from build123d import *

# Parameters (mm, degrees)
BOSS_EXTRUDE1_DEPTH = 7.62


with BuildPart() as part:
    # Sketch1 → Revolve1 (revolve)
    with BuildSketch(Plane.XY):
        Polygon((0, 1.778), (0, 2.54), (0.635, 2.54), (0.635, 2.032), (7.366, 2.032), (7.366, 2.54), (7.62, 2.54), (7.62, 1.778), (0.635, 1.778), (0.635, 0), (0, 0), align=None)
    revolve(axis=Axis((0, 0, 0), (1, 0, 0)))

    # Sketch3 → Boss-Extrude1 (add)
    with BuildSketch(Plane(origin=(0, 0, 0), x_dir=(0, 0, -1), z_dir=(1, 0, 0))):
        with BuildLine():
            Line((-1.524, 0.762), (-0.762, 0.762))
            Line((-0.762, 0.762), (-0.762, 1.524))
            ThreePointArc((-0.762, 1.524), (0, 2.286), (0.762, 1.524))
            Line((0.762, 1.524), (0.762, 0.762))
            Line((0.762, 0.762), (1.524, 0.762))
            ThreePointArc((1.524, 0.762), (2.286, 0), (1.524, -0.762))
            Line((1.524, -0.762), (0.762, -0.762))
            Line((0.762, -0.762), (0.762, -1.524))
            ThreePointArc((0.762, -1.524), (0, -2.286), (-0.762, -1.524))
            Line((-0.762, -1.524), (-0.762, -0.762))
            Line((-0.762, -0.762), (-1.524, -0.762))
            ThreePointArc((-1.524, -0.762), (-2.286, 0), (-1.524, 0.762))
        make_face()
    extrude(amount=-BOSS_EXTRUDE1_DEPTH)


solid = part.part
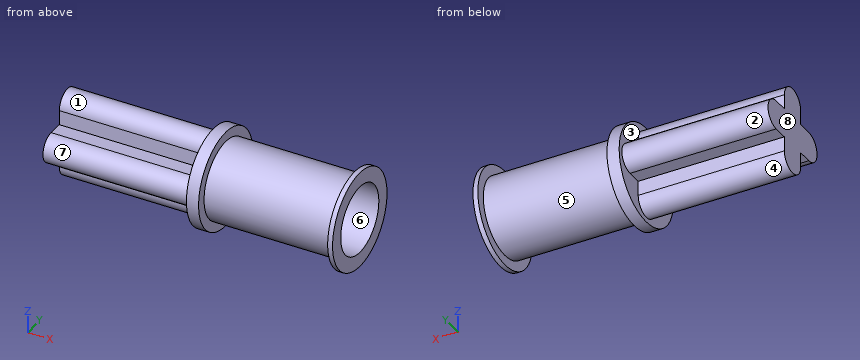
CAD build for the part. Positions are in the model's coordinates, mm. Face numbers are marked on the shaded views. A direction names the side the tool comes from. Round coordinates to 2 decimals unless told otherwise and drop trailing zeros. Write each loop counter-clockwise with the first axis right and the second up, starting at its lowest first coordinate (ties: lowest second). Pieces come first, ordered by that corner, then holes. Notation, with made-up numbers: M 55.25,54.25 L 75.25,54.25 A34 ccw 75.25,89.25 Z; hole C -17,7 d4. An arc over 180 degrees is marked long. Use a Markdown table: item, result. Add a question column.
1. Slice it at B-B on x = -4. Give the cut face in (y, z), then the cut area to 3 significant figures.
2. Slice it at D-D on x = 4. Give the cut face in (y, z), then the cut area to 3 significant figures.
3. Drill centre lines: probe 1 along X at (y, z) = (-2.15, 0.95) (3 decimals); probe 2 along Z at (x, y) = (-1.25, -1.1); probe 3 along X at (y, z) = (-0.7, -0.3) (3 decimals). Where is each one in solid material? Low to high.
4. 3-axis set-ups, long thin cutter, end or side, ignore diameter. For the marked faces 1, 2, 3, 4 and 5: which of +Z, -Z, +X, -X, +Y, -Y reach the whole face in a straight line?
5. Slice it at A-A on z = 0. Give the cut face in (x, y) (3 decimals).
6. Flat gauge pins, fed straight in: P1, Ø3, axis at x = 5, y = -1.5, coming from the -Z side; P2, Ø0.8, axis at x = -3.5, y = 1.5, coming from the -Z side; P3, Ø1.5, axis at x = -1, y = 0.5, coming from the +Z side. Where does each tip first touch, or does it go through?
7. Pull direction Y, two halves, no side cores. Call the marked faces 6, 7 and 8: released by +Y, released by -Y, zero draft, split by the parting line, or undercut.
Reply:
| question | item | result |
|---|---|---|
| 1 | outline | M -1.52,-0.76 L -0.76,-0.76 L -0.76,-1.52 A0.76 ccw 0.76,-1.52 L 0.76,-0.76 L 1.52,-0.76 A0.76 ccw 1.52,0.76 L 0.76,0.76 L 0.76,1.52 A0.76 ccw -0.76,1.52 L -0.76,0.76 L -1.52,0.76 A0.76 ccw Z |
| 1 | area | 10.6 mm^2 |
| 2 | outline | C 0,0 d4.06; hole C 0,0 d3.56 |
| 2 | area | 3.04 mm^2 |
| 3 | probe 1 | x = 0 to 0.635, 7.366 to 7.62 |
| 3 | probe 2 | z = -0.76 to 0.76 |
| 3 | probe 3 | x = -7.62 to 0.635 |
| 4 | face 1 | +Z, -X |
| 4 | face 2 | -X, +Y |
| 4 | face 3 | -X |
| 4 | face 4 | -Z, -X |
| 4 | face 5 | none |
| 5 | outline | M -7.62,-2.286 L 0,-2.286 L 0,-2.54 L 0.635,-2.54 L 0.635,-2.032 L 7.366,-2.032 L 7.366,-2.54 L 7.62,-2.54 L 7.62,-1.778 L 0.635,-1.778 L 0.635,1.778 L 7.62,1.778 L 7.62,2.54 L 7.366,2.54 L 7.366,2.032 L 0.635,2.032 L 0.635,2.54 L 0,2.54 L 0,2.286 L -7.62,2.286 Z |
| 6 | P1 | stops at z = -2.03 |
| 6 | P2 | stops at z = -0.76 |
| 6 | P3 | stops at z = 2.29 |
| 7 | face 6 | undercut |
| 7 | face 7 | released by -Y |
| 7 | face 8 | zero draft |
